from build123d import *

# Parameters (mm, degrees)
F0_W     = 90.371005
F0_H     = 139.010184
F1_DEPTH = 2.54
F2_T     = -2.54
F3_R     = 14.428141
F4_DEPTH = 22.606


with BuildPart() as f1:
    # F0 (on Top) → F1 (new body)
    with BuildSketch(Plane.XY):
        with Locations((-13.526871, -9.353686)):
            Rectangle(F0_W, F0_H)
    extrude(amount=-F1_DEPTH)

    # F2
    f2_openings = [f1.faces().sort_by_distance(p)[0] for p in [
        (-13.526872, -9.353686, 0),
    ]]
    offset(amount=F2_T, openings=f2_openings)

    # F3 (on face) → F4 (join)
    with BuildSketch(Plane.XY):
        with Locations((-13.762863, 36.496103)):
            Circle(F3_R)
    extrude(amount=F4_DEPTH)


solid = f1.part
Design review of the part built by this model. Coordinates are the model's own, in mm. Give positions to 0.01 mm unless a question says otherwise; leave off trailing zeros. Loops run counter-clockwise (first coordinate to the right, second up) from the corner with the lowest first, then second, coordinate; pieces in that order, holes last. Notation, with made-up numbers: (71, 39.25) - (85, 39.25) arc R5 cw to (85, 46.25) - close; hole circle Ø10 at (24.5, -32.75). An arc over 180 degrees is marked (long way). Use CSV: the item, a comma, the result in double quotes. Start each with the question number.
1. Add section A-A (x = -9). State the section outline as (y, z) points, plus the area to 3 significant figures.
2. Add section D-D (y = -25.5). State the section outline as (x, z) points.
3. Add section B-B (y = 42). State the section outline as (x, z) points.
4. Wall thickness on L1, parallel to Z at x = 25, y = 11.5; L2, parallel to Y at x = -24, z = 11.5; L3, parallel to Y at x = -19.5, z = 2.5: over which ranges is each line inside the solid? List them lowest first.
5. Insertion check: P1, Ø3, axis at x = -14, z = 7, coming from the -Y side; P2, Ø3, axis at x = -18, z = 14, coming from the +Y side; P3, Ø6, axis at x = -15.5, z = 10, coming from the +Y side. Each pin has a flat end and moves straight along its axis. Give the tip position at first contact, or say it passes through.
6. Draft analysis for pull direction Y (two halves, no side actions). For faces 1 (the flat face through (-14, -78.859, -1)), 2 (the flat face through (-58.712, -10, -1)), 3 (the flat face through (-14, 60.151, -1)), 4 (the cylindrical face through (-7.1, 23.7, 11.1)), state which applies: released by +Y, released by -Y, zero draft, split by the parting line, or undercut.
7. Add section C-C (x = -53). State the section outline as (y, z) points, plus the area to 3 significant figures.
Results found:
1,outline,"(-78.86, -2.54) - (60.15, -2.54) - (60.15, 0) - (50.12, 0) - (50.12, 22.61) - (22.88, 22.61) - (22.88, 0) - (-78.86, 0) - close"
1,area,"969 mm²"
2,outline,"(-58.71, -2.54) - (31.66, -2.54) - (31.66, 0) - (-58.71, 0) - close"
3,outline,"(-58.71, -2.54) - (31.66, -2.54) - (31.66, 0) - (-0.43, 0) - (-0.43, 22.61) - (-27.1, 22.61) - (-27.1, 0) - (-58.71, 0) - close"
4,L1,"z = -2.54 to 0"
4,L2,"y = 26.33 to 46.66"
4,L3,"y = 23.26 to 49.73"
5,P1,"stops at y = 22.07"
5,P2,"stops at y = 50.66"
5,P3,"stops at y = 50.92"
6,face 1,"released by -Y"
6,face 2,"zero draft"
6,face 3,"released by +Y"
6,face 4,"split by the parting line"
7,outline,"(-78.86, -2.54) - (60.15, -2.54) - (60.15, 0) - (-78.86, 0) - close"
7,area,"353 mm²"
